from build123d import *

# Parameters (mm, degrees)
SKETCH_1_W      = 6.1
SKETCH_1_H      = 7.5
EXTRUDE_1_DEPTH = 3.6
SKETCH_1_3_R    = 1.8
EXTRUDE_2_DEPTH = 10.1
EXTRUDE_START   = 3.6
SKETCH_1_4_R    = 0.5
EXTRUDE_3_DEPTH = 0.3
SKETCH_2_W      = 0.8
SKETCH_2_H      = 0.4
EXTRUDE_4_DEPTH = 4.4
EXTRUDE_START_2 = -6.1
SKETCH_4_W      = 0.5
SKETCH_4_H      = 6.4
EXTRUDE_5_DEPTH = 7
SKETCH_4_3_W    = 0.5
SKETCH_4_3_H    = 1
EXTRUDE_6_DEPTH = 4.4


with BuildPart() as part:
    # 草图1 → 凸台-拉伸1 (new body)
    with BuildSketch(Plane(origin=(0, 0, 0), x_dir=(1, 0, 0), z_dir=(0, 1, 0))):
        Rectangle(SKETCH_1_W, SKETCH_1_H)
    extrude(amount=EXTRUDE_1_DEPTH)

    # 草图1<3> → 凸台-拉伸2 (add)
    with BuildSketch(Plane(origin=(0, 0, 0), x_dir=(1, 0, 0), z_dir=(0, 1, 0))):
        with Locations(Location((0, 0, 0), (0, 0, 90))):
            Circle(SKETCH_1_3_R)
    extrude(amount=EXTRUDE_2_DEPTH)

    # 草图1<4> → 凸台-拉伸3 (add)
    with BuildSketch(Plane(origin=(0, 0, 0), x_dir=(1, 0, 0), z_dir=(0, 1, 0)).offset(EXTRUDE_START)):
        with Locations(Location((-1.708, 2.1, 0), (0, 0, 90))):
            Circle(SKETCH_1_4_R)
        with Locations(Location((-1.708, -2.1, 0), (0, 0, 90))):
            Circle(SKETCH_1_4_R)
        with Locations(Location((1.708, -2.1, 0), (0, 0, 90))):
            Circle(SKETCH_1_4_R)
        with Locations(Location((1.708, 2.1, 0), (0, 0, 90))):
            Circle(SKETCH_1_4_R)
    extrude(amount=EXTRUDE_3_DEPTH)

    # 草图2 → 凸台-拉伸4 (add)
    with BuildSketch(Plane(origin=(3.05, 0, 0), x_dir=(0, 0, -1), z_dir=(1, 0, 0))):
        with Locations((-2.2, 1.1)):
            Rectangle(SKETCH_2_W, SKETCH_2_H)
        with Locations((2.2, 1.1)):
            Rectangle(SKETCH_2_W, SKETCH_2_H)
    extrude(amount=EXTRUDE_4_DEPTH)

    # 草图4 → 凸台-拉伸5 (add)
    with BuildSketch(Plane(origin=(3.05, 0, 0), x_dir=(0, 0, -1), z_dir=(1, 0, 0)).offset(EXTRUDE_START_2)):
        with Locations((-3.5, 0.4)):
            Rectangle(SKETCH_4_W, SKETCH_4_H)
        with Locations((3.5, 0.4)):
            Rectangle(SKETCH_4_W, SKETCH_4_H)
    extrude(amount=EXTRUDE_5_DEPTH)

    # 草图4<3> → 凸台-拉伸6 (add)
    with BuildSketch(Plane(origin=(3.05, 0, 0), x_dir=(0, 0, -1), z_dir=(1, 0, 0))):
        with Locations((3.5, -1.3)):
            Rectangle(SKETCH_4_3_W, SKETCH_4_3_H)
        with Locations((-3.5, -1.3)):
            Rectangle(SKETCH_4_3_W, SKETCH_4_3_H)
    extrude(amount=EXTRUDE_6_DEPTH)


solid = part.part
Design review of the part built by this model. Coordinates are the model's own, in mm. A direction names the side the tool comes from. Coordinates: 2 decimals unless noted, no trailing zeros. Order: outer loops, then holes, each group sorted by start corner. A loop starts at its lowest first (then second) coordinate and runs counter-clockwise, first axis right, second up.
Item 1: Take a section at B-B, the plane x = 3.75. Write out the cut boundary in (y, z).
Item 2: For faces 1 (the flat face through (-2, 3.9, 2)), 2 (the flat face through (2, 3.6, 0)), 3 (the flat face through (2, -1, -3.25)), 4 (the flat face through (2, 3.9, 2)), 5 (the flat face through (-2, 3.9, -2)), list the 3-axis set-ups (+Z, -Z, +X, -X, +Y, -Y) from which the entire face can be reached by the end or side of a thin tool; tool diameter is ignored.
Item 3: For pin 1 Ø0.8 at (x, z) = (2, -2) entering from +Y; pin 2 Ø4 at (y, z) = (5, 3) entering from +X, all flat-tipped, find the tip position at first contact; note any pin that passes through.
Item 4: Take a section at A-A, the plane y = -1. Write out the cut boundary in (x, z).
Item 5: For line 1 (Z direction, x = 3, y = -2); line 2 (X direction, y = 2.25, z = 2.5); line 3 (Y direction, x = -2.25, z = -3.5), list the stretches that pass through material, from the lowest coordinate up.
Item 6: Take a section at D-D, the plane x = 0. Write out the cut boundary in (y, z).
Item 7: Take a section at C-C, the plane z = 0. Write out the cut boundary in (x, y).
Item 8: The part is to be moulded in two halves that separate along Z. For faces 6 (the flat face through (2, -1, 3.25)), 7 (the flat face through (2, 3.9, -2)), 8 (the flat face through (1, 0, 3.75)), 9 (the flat face through (0, 0, 0)), say which applies: pulls with the +Z half, pulls with the -Z half, needs draft (parallel to the pull), parting line crosses it, or undercut.
The answers:
1. outline: (-2.8, -3.75) - (3.6, -3.75) - (3.6, -3.25) - (-2.8, -3.25) - close; (-2.8, 3.25) - (3.6, 3.25) - (3.6, 3.75) - (-2.8, 3.75) - close; (0.9, -2.6) - (1.3, -2.6) - (1.3, -1.8) - (0.9, -1.8) - close; (0.9, 1.8) - (1.3, 1.8) - (1.3, 2.6) - (0.9, 2.6) - close
2. face 1: +Z, -X, +Y
2. face 2: +Y
2. face 3: +X, -Y
2. face 4: +Z, +X, +Y
2. face 5: -Z, -X, +Y
3. pin 1: stops at y = 3.9
3. pin 2: stops at x = 3.95
4. outline: (-3.05, -3.75) - (7.45, -3.75) - (7.45, -3.25) - (-3.05, -3.25) - close; (-3.05, 3.25) - (7.45, 3.25) - (7.45, 3.75) - (-3.05, 3.75) - close
5. line 1: z = -3.75 to -3.25, 3.25 to 3.75
5. line 2: x = -3.05 to 3.05
5. line 3: y = -2.8 to 3.6
6. outline: (-2.8, -3.75) - (3.6, -3.75) - (3.6, -1.8) - (10.1, -1.8) - (10.1, 1.8) - (3.6, 1.8) - (3.6, 3.75) - (-2.8, 3.75) - (-2.8, 3.25) - (0, 3.25) - (0, -3.25) - (-2.8, -3.25) - close
7. outline: (-3.05, 0) - (3.05, 0) - (3.05, 3.6) - (1.8, 3.6) - (1.8, 10.1) - (-1.8, 10.1) - (-1.8, 3.6) - (-3.05, 3.6) - close
8. face 6: undercut
8. face 7: needs draft
8. face 8: pulls with the +Z half
8. face 9: undercut
